from build123d import *

# Parameters (mm, degrees)
SKETCH_1_R          = 12.9
SKETCH_1_R_2        = 11.1
EXTRUDE_1_DEPTH     = 5
SKETCH_3_R          = 16.662816376
SKETCH_3_R_2        = 12
CUT_EXTRUDE_1_DEPTH = 4
CHAMFER_1_SIZE      = 0.5


with BuildPart() as part:
    # 草图1 → 凸台-拉伸1 (new body)
    with BuildSketch(Plane.XY):
        Circle(SKETCH_1_R)
        Circle(SKETCH_1_R_2, mode=Mode.SUBTRACT)
    extrude(amount=EXTRUDE_1_DEPTH)

    # 草图3 → 切除-拉伸1 (cut)
    with BuildSketch(Plane.XY.offset(5)):
        Circle(SKETCH_3_R)
        Circle(SKETCH_3_R_2, mode=Mode.SUBTRACT)
    extrude(amount=-CUT_EXTRUDE_1_DEPTH, mode=Mode.SUBTRACT)

    # 倒角1
    chamfer_1_edges = [part.edges().sort_by_distance(p)[0] for p in [
        (-12, 0, 5),
    ]]
    chamfer(chamfer_1_edges, length=CHAMFER_1_SIZE)


solid = part.part
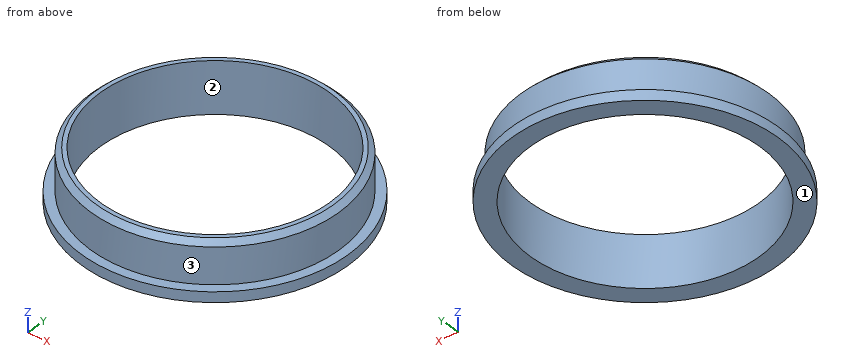
Here's how the part is built. I have some questions about the finished solid (model axes, mm). Face numbers are marked on the shaded views. Round coordinates to 2 decimals unless told otherwise and drop trailing zeros. Loops run counter-clockwise (first coordinate to the right, second up) from the corner with the lowest first, then second, coordinate; pieces in that order, holes last. Notation, with made-up numbers: (12.5, 2.25) -> (41.5, 2.25) arc R36 ccw to (41.5, 39.25) -> close; hole circle Ø4 at (78.5, -4). An arc over 180 degrees is marked (long way). Write each question's results on one line, items separated by ' | '.
(1) For P1, Ø10, axis at x = 0.5, y = -10, coming from the -Z side; P2, Ø3, axis at x = 8.5, z = 3.5, coming from the +Y side, each with a flat end and sliding along its axis, tell me the tip position at first contact or that it passes through.
Worked answers:
P1: z = 0 | P2: y = 9.75
(2) If we section it at A-A, the plane x = 0: List the corners of the cut face in (y, z) for me.
Worked answers:
outline: (-12.9, 0) -> (-11.1, 0) -> (-11.1, 5) -> (-11.5, 5) -> (-12, 4.5) -> (-12, 1) -> (-12.9, 1) -> close; (11.1, 0) -> (12.9, 0) -> (12.9, 1) -> (12, 1) -> (12, 4.5) -> (11.5, 5) -> (11.1, 5) -> close
(3) If we section it at C-C, the plane z = 1.45: List the corners of the cut face in (x, y) for me.
Worked answers:
outline: circle Ø24 at (0, 0); hole circle Ø22.2 at (0, 0)
(4) We'd pull the mould along Y, two halves only. Please class the marked faces 1, 2 and 3: released by +Y, released by -Y, zero draft, split by the parting line, or undercut.
Worked answers:
face 1: zero draft | face 2: undercut | face 3: split by the parting line
(5) If I drill on L1, parallel to Y at x = 0, z = 3.05; L2, parallel to Z at x = 10.5, y = -6.25; L3, parallel to X at y = 10, z = 0.55, over which ranges is the centre line in solid material (lowest first)?
Worked answers:
L1: -12 to -11.1, 11.1 to 12 | L2: 0 to 1 | L3: -8.15 to -4.82, 4.82 to 8.15
